```python
from build123d import *

# Parameters (mm, degrees)
F0_W     = 71
F0_H     = 36
F1_DEPTH = 2
F3_DEPTH = 6.8
F4_R     = 2
F5_R     = 1.25
F6_DEPTH = 8.801
F7_R     = 1.5
F8_DEPTH = 33.501
F9_SIZE  = 1


with BuildPart() as f1:
    # F0 (on Top) → F1 (new body)
    with BuildSketch(Plane.XY):
        with Locations((35.5, -18)):
            Rectangle(F0_W, F0_H)
    extrude(amount=F1_DEPTH)

    # F2 (on face) → F3 (join)
    with BuildSketch(Plane.XY.offset(2)):
        Polygon((25.5, -2.5), (2.5, -2.5), (2.5, -33.5), (68.5, -33.5), (68.5, -2.5), (62.5, -2.5), (62.5, -3.5), (67.5, -3.5), (67.5, -32.5), (3.5, -32.5), (3.5, -3.5), (25.5, -3.5), align=None)
    extrude(amount=F3_DEPTH)

    # F4
    f4_edges = [f1.edges().sort_by_distance(p)[0] for p in [
        (0, -36, 1),
        (0, 0, 1),
        (71, -36, 1),
        (71, 0, 1),
    ]]
    fillet(f4_edges, radius=F4_R)

    # F5 (on face) → F6 (cut, through all)
    with BuildSketch(Plane(origin=(0, 0, 0), x_dir=(1, 0, 0), z_dir=(0, 0, -1))):
        with Locations((16.25, 29.75)):
            Circle(F5_R)
        with Locations((19.25, 29.75)):
            Circle(F5_R)
    extrude(amount=-F6_DEPTH, mode=Mode.SUBTRACT)

    # F7 (on face) → F8 (cut, through all)
    with BuildSketch(Plane(origin=(0, -2.5, 0), x_dir=(-1, 0, 0), z_dir=(0, 1, 0))):
        with Locations((-64.7, 5)):
            Circle(F7_R)
        with Locations((-6.3, 5)):
            Circle(F7_R)
    extrude(amount=-F8_DEPTH, mode=Mode.SUBTRACT)

    # F9
    f9_edges = [f1.edges().sort_by_distance(p)[0] for p in [
        (2.5, -2.5, 5.4),
        (68.5, -33.5, 5.4),
        (68.5, -2.5, 5.4),
        (2.5, -33.5, 5.4),
    ]]
    chamfer(f9_edges, length=F9_SIZE)


solid = f1.part
```
Model file for the job. Use its own axes, mm. A direction names the side the tool comes from. Give positions to 0.01 mm unless a question says otherwise; leave off trailing zeros. Write each loop counter-clockwise with the first axis right and the second up, starting at its lowest first coordinate (ties: lowest second). Pieces come first, ordered by that corner, then holes. Notation, with made-up numbers: (-19.75, -25.5) -> (-11.75, -25.5) arc R20 cw to (-11.75, -5.5) -> close; hole circle Ø1 at (44.5, 64.5). An arc over 180 degrees is marked (long way). Use CSV: the item, a comma, the result in double quotes. Start each with the question number.
1) Cut at A-A on x = 64.7. List the corners of the cut face in (y, z).
2) Tool access for faces 1 (the cylindrical face through (4.87, -32.99, 5.45)), 2 (the flat face through (36, -32.5, 5)), 3 (the flat face through (15, -2.5, 5)), 4 (the flat face through (35, 0, 1)), 5 (the flat face through (68.5, -18, 5)): list every direction of +Z, -Z, +X, -X, +Y, -Y with a clear straight run to the whole face (end or side of a thin tool).
3) Cut at C-C on y = -20. List the corners of the cut face in (x, z).
4) Two-plate mould, pull along X, no slides. Class faces 6 (the flat face through (35, -33.5, 5)), 7 (the cylindrical face through (64.01, -32.99, 3.67)), 8 (the flat face through (2.5, -18, 5)): released by +X, released by -X, zero draft, split by the parting line, or undercut.
5) Cut at D-D on x = 52.5. List the corners of the cut face in (y, z), plus the area to 3 significant figures.
6) Pin check, flat tips, straight feed: P1, Ø3.5, axis at x = 39.5, z = 5.5, coming from the -Y side; P2, Ø2, axis at y = -19, z = 6, coming from the +X side; P3, Ø3.5, axis at x = 29.5, z = 4, coming from the +Y side. Stop position of each tip, or through.
7) Drill centre lines: L1, parallel to Y at x = 5, z = 4; L2, parallel to Z at x = 6.3, y = -32.75; L3, parallel to X at y = -6.5, z = 8.5. Where is each one in solid material? Low to high.
8) Cut at B-B on x = 16.25. List the corners of the cut face in (y, z).
Final values:
1,outline,"(-36, 0) -> (0, 0) -> (0, 2) -> (-2.5, 2) -> (-2.5, 3.5) -> (-3.5, 3.5) -> (-3.5, 2) -> (-32.5, 2) -> (-32.5, 3.5) -> (-33.5, 3.5) -> (-33.5, 2) -> (-36, 2) -> close; (-33.5, 6.5) -> (-32.5, 6.5) -> (-32.5, 8.8) -> (-33.5, 8.8) -> close; (-3.5, 6.5) -> (-2.5, 6.5) -> (-2.5, 8.8) -> (-3.5, 8.8) -> close"
2,face 1,"+Y, -Y"
2,face 2,"+Z"
2,face 3,"+Z, +X, -X, +Y"
2,face 4,"+Z, -Z, +X, -X, +Y"
2,face 5,"+Z, +X, +Y, -Y"
3,outline,"(0, 0) -> (71, 0) -> (71, 2) -> (68.5, 2) -> (68.5, 8.8) -> (67.5, 8.8) -> (67.5, 2) -> (3.5, 2) -> (3.5, 8.8) -> (2.5, 8.8) -> (2.5, 2) -> (0, 2) -> close"
4,face 6,"zero draft"
4,face 7,"undercut"
4,face 8,"released by -X"
5,outline,"(-36, 0) -> (0, 0) -> (0, 2) -> (-32.5, 2) -> (-32.5, 8.8) -> (-33.5, 8.8) -> (-33.5, 2) -> (-36, 2) -> close"
5,area,"78.8 mm2"
6,P1,"stops at y = -33.5"
6,P2,"stops at x = 68.5"
6,P3,"stops at y = -32.5"
7,L1,"y = -33.5 to -32.5, -3.5 to -2.5"
7,L2,"z = 0 to 3.5, 6.5 to 8.8"
7,L3,"x = 2.5 to 3.5, 67.5 to 68.5"
8,outline,"(-36, 0) -> (-31, 0) -> (-31, 2) -> (-32.5, 2) -> (-32.5, 8.8) -> (-33.5, 8.8) -> (-33.5, 2) -> (-36, 2) -> close; (-28.5, 0) -> (0, 0) -> (0, 2) -> (-2.5, 2) -> (-2.5, 8.8) -> (-3.5, 8.8) -> (-3.5, 2) -> (-28.5, 2) -> close"
